Can you work these out from the drawing? Everything is in mm from the part's minimum corner. A direction names the side the tool comes from. Coordinates: 2 decimals unless noted, no trailing zeros. Loops run counter-clockwise (first coordinate to the right, second up) from the corner with the lowest first, then second, coordinate; pieces in that order, holes last. Notation, with made-up numbers: M 8,82 L 62,82 A19 ccw 62,96 Z; hole C 35.5,-32 d7. An arc over 180 degrees is marked long. Use CSV: the item, a comma, the result in double quotes. Start each with the question number.
Q1. If we section it at D-D (x = 20.5): Please give me the cut outline in (y, z).
Q2. Which directions (+Z, -Z, +X, -X, +Y, -Y) give clear straight access to the entire face, cutting with the end or side of a thin tool? Please do the marked faces 1 and 2.
Q3. If we section it at A-A (y = 20): Please give me the cut outline in (x, z).
Q4. Please list where these lines run through material, in increasing order: probe 1 along X at (y, z) = (1.05, 5); probe 2 along X at (y, z) = (25, 32.5). Write a range as [from, to].
Q5. For pin 1 Ø1.9 at (y, z) = (12.58, 27.75) entering from +X; pin 2 Ø4.5 at (x, z) = (9.5, 35) entering from +Y; pin 3 Ø4 at (y, z) = (26, 35.5) entering from +X; pin 4 Ø1.6 at (x, y) = (1, 28) entering from -Z, each with a flat end and sliding along its axis, tell me the tip position at first contact or that it passes through.
Q6. If we section it at C-C (z = 35): Please give me the cut outline in (x, y), and give its area (3 significant figures).
Q7. If we section it at B-B (z = 27.5): Please give me the cut outline in (x, y).
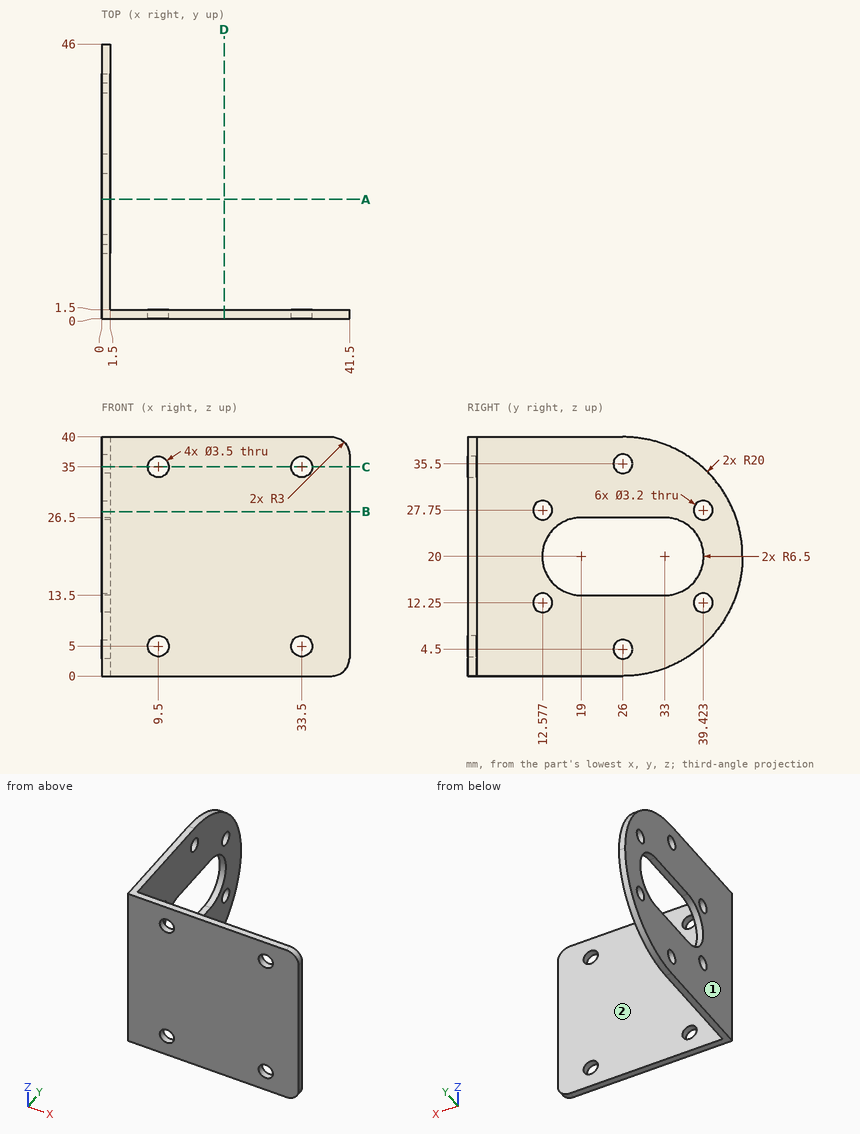
Results below:
1,outline,"M 0,0 L 1.5,0 L 1.5,40 L 0,40 Z"
2,face 1,"+Z, -Z, -X, +Y, -Y"
2,face 2,"+Z, -Z, +X, +Y"
3,outline,"M 0,0 L 1.5,0 L 1.5,13.5 L 0,13.5 Z; M 0,26.5 L 1.5,26.5 L 1.5,40 L 0,40 Z"
4,probe 1,"[0, 7.75], [11.25, 31.75], [35.25, 41.5]"
4,probe 2,"[0, 1.5]"
5,pin 1,"through"
5,pin 2,"y = 1.5"
5,pin 3,"x = 1.5"
5,pin 4,"z = 0.04"
6,outline,"M 0,0 L 7.75,0 L 7.75,1.5 L 1.5,1.5 L 1.5,24.48 L 0,24.48 Z; M 0,27.52 L 1.5,27.52 L 1.5,39.23 L 0,39.23 Z; M 11.25,0 L 31.75,0 L 31.75,1.5 L 11.25,1.5 Z; M 35.25,0 L 41.5,0 L 41.5,1.5 L 35.25,1.5 Z"
6,area,"104 mm^2"
7,outline,"M 0,0 L 41.5,0 L 41.5,1.5 L 1.5,1.5 L 1.5,11 L 0,11 Z; M 0,14.16 L 1.5,14.16 L 1.5,37.84 L 0,37.84 Z; M 0,41 L 1.5,41 L 1.5,44.54 L 0,44.54 Z"
